Autodesk Inventor part; units mm, degrees
ref_plane "YZ Plane" through (0, 0, 0) normal (1, 0, 0) x (0, 1, 0)
ref_plane "XZ Plane" through (0, 0, 0) normal (0, 1, 0) x (-1, 0, 0)
ref_plane "XY Plane" through (0, 0, 0) normal (0, 0, 1) x (1, 0, 0)
sketch "Sketch1" plane through (0, 0, 0) normal (0, 0, 1) x (1, 0, 0)
  line L0 (0, 0) -> (76.2, 0)
  arc A0 (0, 0) -> (0, -38.1) centre (0, -19.05) ccw
  arc A1 (76.2, -38.1) -> (76.2, 0) centre (76.2, -19.05) ccw
  line L1 (76.2, -38.1) -> (63.5, -38.1)
  line L2 (0, -38.1) -> (12.7, -38.1)
  arc A2 (21.4597, -48.4605) -> (12.7, -38.1) centre (12.7, -46.9833) ccw
  arc A3 (21.4597, -48.4605) -> (22.5109, -60.7745) centre (45.8763, -52.578) ccw
  arc A4 (22.5109, -60.7745) -> (25.5069, -62.8985) centre (25.5069, -59.7235) ccw
  line L3 (25.5069, -62.8985) -> (50.6931, -62.8985)
  circle A5 centre (0, -19.05) radius 1.778
  circle A6 centre (76.2, -19.05) radius 1.778
  line L4 (-19.05, -19.05) -> (-19.05, 0)
  line L5 (95.25, -19.05) -> (95.25, 0)
  line L6 (30.3237, -52.578) -> (45.8763, -52.578)
  circle A7 centre (38.1, -46.228) radius 1.778
  circle A8 centre (38.1, -58.928) radius 1.778
  arc A9 (63.5, -38.1) -> (54.7403, -48.4605) centre (63.5, -46.9833) ccw
  arc A10 (53.6891, -60.7745) -> (54.7403, -48.4605) centre (30.3237, -52.578) ccw
  arc A11 (50.6931, -62.8985) -> (53.6891, -60.7745) centre (50.6931, -59.7235) ccw
  point P0 (23.3871, -62.9395)
  dimension "d0" = 76.2
  dimension "d1" = 38.1
  dimension "d5" = 12.7
  dimension "d6" = 12.7
  dimension "d8" = 3.175
  dimension "d9" = 3.556
  dimension "d10" = 3.556
  dimension "d14" = 19.05
  dimension "d15" = 19.05
  dimension "d16" = 3.556
  dimension "d17" = 6.35
  dimension "d18" = 3.556
  dimension "d19" = 12.7
  dimension "d22" = 6.35
extrude "Extrusion3" add sketch "Sketch1" along normal blind 5.842
properties part number "casing"
Work out the finished part from the listing and answer in its coordinate system (mm). A direction names the side the tool comes from. Give positions to 0.01 mm unless a question says otherwise; leave off trailing zeros. Order: outer loops, then holes, each group sorted by start corner. A loop starts at its lowest first (then second) coordinate and runs counter-clockwise, first axis right, second up.
1. Section B-B, the plane x = 38.1 is taken. Determine the outline of the cut face in (y, z), and give its area (3 significant figures).
Result sheet:
outline: (-62.9, 0) - (-60.71, 0) - (-60.71, 5.84) - (-62.9, 5.84) - close; (-57.15, 0) - (-48.01, 0) - (-48.01, 5.84) - (-57.15, 5.84) - close; (-44.45, 0) - (0, 0) - (0, 5.84) - (-44.45, 5.84) - close
area: 326 mm2
2. The mould has two halves that part along X. Classify faces 4 (the cylindrical face through (-0.231, -20.813, 2.88)), 5 (the cylindrical face through (19.413, -41.166, 2.88)), 6 (the cylindrical face through (38.92, -57.35, 2.88)), 7 (the cylindrical face through (52.55, -62.3, 2.88)): released by +X, released by -X, zero draft, split by the parting line, or undercut.
Result sheet:
face 4: undercut
face 5: released by -X
face 6: undercut
face 7: released by +X
3. Section D-D, the plane x = 72.5 is taken. Determine the outline of the cut face in (y, z), and give its area (3 significant figures).
Result sheet:
outline: (-38.1, 0) - (0, 0) - (0, 5.84) - (-38.1, 5.84) - close
area: 223 mm2
4. For faces 1 (the flat face through (6, -38.1, 3)), 2 (the flat face through (70, -38.1, 3)), 3 (the cylindrical face through (21.212, -54.771, 2.88)), determine the directions among +Z, -Z, +X, -X, +Y, -Y from which every point of the face is accessible in a straight line to the end or side of a thin tool.
Result sheet:
face 1: +Z, -Z, -X, -Y
face 2: +Z, -Z, +X, -Y
face 3: +Z, -Z, -X
5. Each of these flat-tipped pins is pushed along its axis until it touches: P1, Ø1.5, axis at y = -24.5, z = 5, coming from the -X side; P2, Ø2, axis at y = -12, z = 3.5, coming from the -X side; P3, Ø1.8, axis at x = 7, z = 2.5, coming from the -Y side. Where does it stop, or does it pass through?
Result sheet:
P1: stops at x = -18.46
P2: stops at x = -18.06
P3: stops at y = -38.1
6. Straight lines are drawn through the part: L1, parallel to Y at x = 38.1, z = 2.4; L2, parallel to Y at x = 76.2, z = 4.25; L3, parallel to X at y = -18.5, z = 4.05. For each, find the intervals that lie inside material, in ascending order.
Result sheet:
L1: y = -62.9 to -60.71, -57.15 to -48.01, -44.45 to 0
L2: y = -38.1 to -20.83, -17.27 to 0
L3: x = -19.04 to -1.69, 1.69 to 74.51, 77.89 to 95.24
7. Section C-C, the plane z = 3.6 is taken. Give the number of separate pieces and of enclosed holes in the cut face, and give its area (3 significant figures).
Result sheet:
separate pieces: 1
enclosed holes: 4
area: 4,850 mm2
8. Section A-A, the plane y = -19.05 is taken. Determine the outline of the cut face in (x, z).
Result sheet:
outline: (-19.05, 0) - (-1.78, 0) - (-1.78, 5.84) - (-19.05, 5.84) - close; (1.78, 0) - (74.42, 0) - (74.42, 5.84) - (1.78, 5.84) - close; (77.98, 0) - (95.25, 0) - (95.25, 5.84) - (77.98, 5.84) - close
